The listing builds one solid part. Answer for the finished solid, in the listing's coordinates (mm). Face numbers are marked on the shaded views. A direction names the side the tool comes from. Give positions to 0.01 mm unless a question says otherwise; leave off trailing zeros. Loops run counter-clockwise (first coordinate to the right, second up) from the corner with the lowest first, then second, coordinate; pieces in that order, holes last. Notation, with made-up numbers: M 88,-10.75 L 116,-10.75 A20 cw 116,-5.75 Z; hole C -19.5,49 d11. An arc over 180 degrees is marked long. Use one line per item in the form item = value. Start each with the question number.
1. Each of these flat-tipped pins is pushed along its axis until it touches: pin 1 Ø2 at (x, z) = (-10, 0) entering from +Y; pin 2 Ø4.5 at (x, y) = (15.5, 8.65) entering from +Z; pin 3 Ø4.5 at (x, y) = (-15.5, 8.65) entering from -Z; pin 4 Ø1 at (x, z) = (10.5, 2) entering from +Y. Where does it stop, or does it pass through?
2. The part is cut by section C-C (z = 0). Write down the section's boundary in (x, y), and give its area (3 significant figures).
3. The part is cut by section D-D (y = 24.15). Write down the section's boundary in (x, z).
4. The part is cut by section B-B (x = 10). Write down the section's boundary in (y, z).
5. The mould has two halves that part along X. Classify the marked faces 3, 4, 5 and 6: released by +X, released by -X, zero draft, split by the parting line, or undercut.
6. For the marked faces 1 and 2, determine the directions among +Z, -Z, +X, -X, +Y, -Y from which every point of the face is accessible in a straight line to the end or side of a thin tool.
7. The part is cut by section A-A (x = 0). Write down the section's boundary in (y, z), and give its area (3 significant figures).
8. Straight lines are drawn through the part: line 1 (Y direction, x = 15.5, z = -8.2); line 2 (Z direction, x = 4.5, y = 7); line 3 (Y direction, x = -13, z = -3.5). For each, find the intervals that lie inside material, in ascending order. Write a range as from..to.
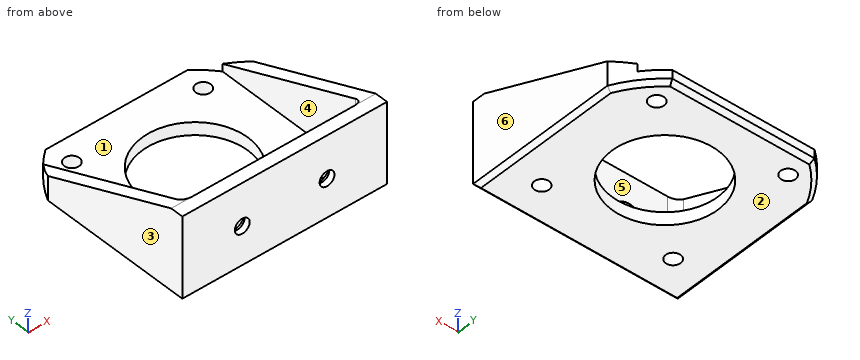
from build123d import *

# Parameters (mm, degrees)
SKETCH1_W           = 48.3
SKETCH1_H           = 20
BOSS_EXTRUDE1_DEPTH = 3
SKETCH2_W           = 48.3
SKETCH2_H           = 3
BOSS_EXTRUDE2_DEPTH = 42.3
SKETCH3_R           = 12.5
SKETCH3_R_2         = 1.75
CUT_EXTRUDE1_DEPTH  = 55.076912819
RIB1_REACH          = 68.97
SKETCH4_WALL_W      = 181.528252596
SKETCH4_WALL_H      = 3
CUT_EXTRUDE2_DEPTH  = 56.093670235
SKETCH6_R           = 1.75
CUT_EXTRUDE3_DEPTH  = 50.724365255
FILLET1_R           = 2
CHAMFER2_SIZE       = 1
CHAMFER3_SIZE       = 1.6


with BuildPart() as part:
    # Sketch1 → Boss-Extrude1 (new body)
    with BuildSketch(Plane(origin=(0, 0, 0), x_dir=(1, 0, 0), z_dir=(0, 1, 0))):
        Rectangle(SKETCH1_W, SKETCH1_H)
    extrude(amount=BOSS_EXTRUDE1_DEPTH)

    # Sketch2 → Boss-Extrude2 (add)
    with BuildSketch(Plane(origin=(0, 3, 0), x_dir=(1, 0, 0), z_dir=(0, 1, 0))):
        with Locations((0, 8.5)):
            Rectangle(SKETCH2_W, SKETCH2_H)
    extrude(amount=BOSS_EXTRUDE2_DEPTH)

    # Sketch3 → Cut-Extrude1 (cut, through all)
    with BuildSketch(Plane.XY.offset(-7)):
        with Locations((0, 24.15)):
            Circle(SKETCH3_R)
        with Locations((-15.5, 39.65)):
            Circle(SKETCH3_R_2)
        with Locations((15.5, 39.65)):
            Circle(SKETCH3_R_2)
        with Locations((15.5, 8.65)):
            Circle(SKETCH3_R_2)
        with Locations((-15.5, 8.65)):
            Circle(SKETCH3_R_2)
    extrude(amount=-CUT_EXTRUDE1_DEPTH, mode=Mode.SUBTRACT)

    # Sketch4 wall → Rib1 (add, up to next)
    with BuildSketch(Plane(origin=(-24.15, 24.15, 1.5), x_dir=(0, -0.927870342081, 0.372902974359), z_dir=(0, 0.372902974359, 0.927870342081)), mode=Mode.PRIVATE) as rib1_sk1:
        with Locations((0, 1.5)):
            Rectangle(SKETCH4_WALL_W, SKETCH4_WALL_H)
    rib1_tool1 = extrude(rib1_sk1.sketch, amount=-RIB1_REACH, mode=Mode.PRIVATE) - part.part
    rib1 = rib1_tool1.solids().sort_by_distance((-24.15, 24.15, 1.5))[0]
    add(rib1)

    # Mirror1: Rib1 across plane
    add(rib1.mirror(Plane(origin=(0, 0, 0), x_dir=(0, 0, 1), z_dir=(1, 0, 0))))

    # Sketch5 → Cut-Extrude2 (cut, through all)
    with BuildSketch(Plane(origin=(0, 0, -10), x_dir=(-1, 0, 0), z_dir=(0, 0, -1))):
        with BuildLine():
            Line((-27, 24.15), (-32.102102735, 24.15))
            ThreePointArc((-32.102102735, 24.15), (0, 56.252102735), (32.102102735, 24.15))
            Line((32.102102735, 24.15), (27, 24.15))
            ThreePointArc((27, 24.15), (0, 51.15), (-27, 24.15))
        make_face()
    extrude(amount=-CUT_EXTRUDE2_DEPTH, mode=Mode.SUBTRACT)

    # Sketch6 → Cut-Extrude3 (cut, through all)
    with BuildSketch(Plane(origin=(0, 3, 0), x_dir=(1, 0, 0), z_dir=(0, 1, 0))):
        with Locations(Location((-10, 0, 0), (0, 0, 270))):
            Circle(SKETCH6_R)
        with Locations(Location((10, 0, 0), (0, 0, 270))):
            Circle(SKETCH6_R)
    extrude(amount=-CUT_EXTRUDE3_DEPTH, mode=Mode.SUBTRACT)

    # Fillet1
    fillet1_edges = [part.edges().sort_by_distance(p)[0] for p in [
        (-21.15, 3, 1.5),
        (21.15, 3, 1.5),
    ]]
    fillet(fillet1_edges, radius=FILLET1_R)

    # Chamfer2
    chamfer2_edges = [part.edges().sort_by_distance(p)[0] for p in [
        (0, 0, -10),
        (0, 45.3, -10),
        (-24.15, 18.111917674, -10),
        (24.15, 18.111917674, -10),
        (20.963705349, 41.165377106, -10),
        (-20.963705349, 41.165377106, -10),
    ]]
    chamfer(chamfer2_edges, length=CHAMFER2_SIZE)

    # Chamfer3
    chamfer3_edges = [part.edges().sort_by_distance(p)[0] for p in [
        (-10, 3, -1.75),
        (10, 3, -1.75),
    ]]
    chamfer(chamfer3_edges, length=CHAMFER3_SIZE)


solid = part.part
Derived:
q1.pin_1 = through
q1.pin_2 = -7
q1.pin_3 = -10
q1.pin_4 = 2.21
q2.outline = M -24.15,0 L -11.75,0 L -11.75,1.4 L -13.35,3 L -19.15,3 A2 cw -21.15,5 L -21.15,27.88 L -24.15,27.88 Z; M -8.25,0 L 8.25,0 L 8.25,1.4 L 6.65,3 L -6.65,3 L -8.25,1.4 Z; M 11.75,0 L 24.15,0 L 24.15,27.88 L 21.15,27.88 L 21.15,5 A2 cw 19.15,3 L 13.35,3 L 11.75,1.4 Z
q2.area = 270 mm2
q3.outline = M -24.15,-9 L -23.15,-10 L -12.5,-10 L -12.5,-7 L -21.15,-7 L -21.15,1.5 L -24.15,1.5 Z; M 12.5,-10 L 23.15,-10 L 24.15,-9 L 24.15,1.5 L 21.15,1.5 L 21.15,-7 L 12.5,-7 Z
q4.outline = M 0,-9 L 1,-10 L 16.65,-10 L 16.65,-7 L 3,-7 L 3,-3.35 L 1.4,-1.75 L 0,-1.75 Z; M 0,1.75 L 1.4,1.75 L 3,3.35 L 3,10 L 0,10 Z; M 31.65,-10 L 44.3,-10 L 45.3,-9 L 45.3,-7 L 31.65,-7 Z
q5.face_3 = released by -X
q5.face_4 = undercut
q5.face_5 = undercut
q5.face_6 = released by +X
q6.face_1 = +Z, +Y
q6.face_2 = -Z, +X, -X, +Y, -Y
q7.outline = M 0,-9 L 1,-10 L 11.65,-10 L 11.65,-7 L 3,-7 L 3,10 L 0,10 Z; M 36.65,-10 L 44.3,-10 L 45.3,-9 L 45.3,-7 L 36.65,-7 Z
q7.area = 111 mm2
q8.line_1 = 0..6.9, 10.4..37.9, 41.4..45.3
q8.line_2 = -10..-7
q8.line_3 = 0..3
